Part model, mm, in its own coordinate system. Face numbers are marked on the shaded views. A direction names the side the tool comes from. Coordinates: 2 decimals unless noted, no trailing zeros. Order: outer loops, then holes, each group sorted by start corner. A loop starts at its lowest first (then second) coordinate and runs counter-clockwise, first axis right, second up.
1) Cut at A-A (y = 0). List the corners of the cut face in (x, z), and give its area (3 significant figures).
2) Wall check: L1, parallel to Z at x = 0.5, y = -9.25; L2, parallel to X at y = 0.25, z = 5.5; L3, parallel to Z at x = -10, y = 8. Give the ranges that are in metal, low to high.
3) Tool access for the marked faces 1 and 2: list every direction of +Z, -Z, +X, -X, +Y, -Y with a clear straight run to the whole face (end or side of a thin tool).
4) Pin check, flat tips, straight feed: pin 1 Ø5 at (x, y) = (3, 7) entering from +Z; pin 2 Ø1.3 at (x, y) = (11.49, -11.49) entering from +Z; pin 3 Ø8 at (y, z) = (10.5, 2) entering from -X; pin 4 Ø2 at (x, y) = (-11.49, -11.49) entering from +Z. Stop position of each tip, or through.
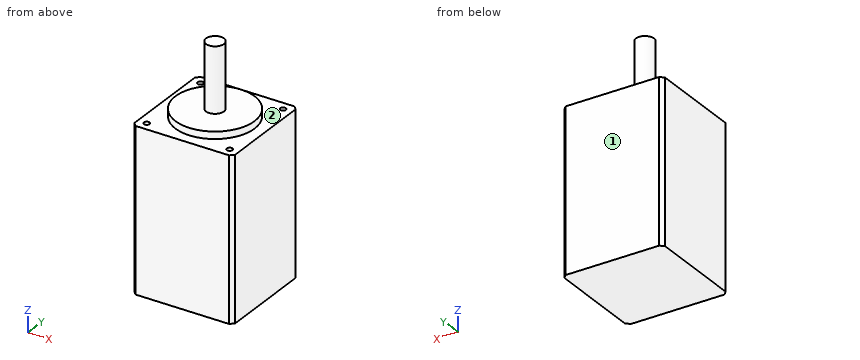
Autodesk Inventor part; units mm, degrees
ref_plane "YZ Plane" through (0, 0, 0) normal (1, 0, 0) x (0, 1, 0)
ref_plane "XZ Plane" through (0, 0, 0) normal (0, 1, 0) x (-1, 0, 0)
ref_plane "XY Plane" through (0, 0, 0) normal (0, 0, 1) x (1, 0, 0)
sketch "Skizze1" plane through (0, 0, 0) normal (0, 0, 1) x (1, 0, 0)
  line L0 (-14, 14) -> (14, 14)
  line L1 (14, 14) -> (14, -14)
  line L2 (14, -14) -> (-14, -14)
  line L3 (-14, -14) -> (-14, 14)
  circle A0 centre (0, 0) radius 11
  circle A1 centre (0, 0) radius 2.5
  line L4 (-14, 0) -> (14, 0) construction
  line L5 (0, 14) -> (0, -14) construction
  line L6 (-11.4905, 11.4905) -> (11.4905, 11.4905) construction
  line L7 (11.4905, 11.4905) -> (11.4905, -11.4905) construction
  line L8 (11.4905, -11.4905) -> (-11.4905, -11.4905) construction
  line L9 (-11.4905, -11.4905) -> (-11.4905, 11.4905) construction
  circle A2 centre (0, 0) radius 16.25 construction
  point P0 (0, -11.4905)
  point P1 (11.4905, 0)
  dimension "d4" = 32.5
  dimension "d0" = 5
  dimension "d1" = 22
  dimension "d2" = 28
extrude "Extrusion1" add sketch "Skizze1" along normal blind 2 contours A0 | A1
extrude "Extrusion2" add sketch "Skizze1" along normal blind 20 contours A1
extrude "Extrusion3" add sketch "Skizze1" against normal blind 45 contours L0 L1 L2 L3 | A0 | A1
hole "Bohrung1" at (-11.4905, 11.4905, 0) at (11.4905, 11.4905, 0) at (11.4905, -11.4905, 0) at (-11.4905, -11.4905, 0) direction (0, 0, -1) diameter 1.567 depth 8 tip angle 118
chamfer "Fase1" distance 1 angle 45 4 edges at (14, -14, -22.5) (-14, -14, -22.5) (14, 14, -22.5) (-14, 14, -22.5)
properties part number "Nema11" material "Stahl"
Geometry check:
1. outline: (-14, -45) - (14, -45) - (14, 0) - (11, 0) - (11, 2) - (2.5, 2) - (2.5, 20) - (-2.5, 20) - (-2.5, 2) - (-11, 2) - (-11, 0) - (-14, 0) - close
1. area: 1,390 mm2
2. L1: z = -45 to 2
2. L2: x = -2.49 to 2.49
2. L3: z = -45 to 0
3. face 1: +Z, -Z, +X, -X, +Y
3. face 2: +Z
4. pin 1: stops at z = 2
4. pin 2: stops at z = -8.08
4. pin 3: stops at x = -14
4. pin 4: stops at z = 0
